The model under review builds one solid part; all positions refer to its coordinate system, in mm. Round coordinates to 2 decimals unless told otherwise and drop trailing zeros. Use CSV: the item, a comma, the result in double quotes. Start each with the question number.
1) For pin 1 Ø4 at (x, y) = (-155, 0) entering from -Z; pin 2 Ø1.5 at (y, z) = (3.5, -1) entering from +X, all flat-tipped, find the tip position at first contact; note any pin that passes through.
2) Mouldability with a two-part tool opening along Y and no side actions: class faces 1 (the face through (-2, 2, -3)), 2 (the face through (-2, -7.5, 0)), 3 (the face through (157.385, 0.751, -0.042)) as released by +Y, released by -Y, zero draft, split by the parting line, or undercut.
3) Wall thickness on probe 1 along Y at (x, z) = (-155, 0.9); probe 2 along X at (y, z) = (-1.25, 1); probe 3 along X at (y, z) = (1, 2.25): over which ranges is each line inside the solid? List them lowest first. Write a range as [from, to].
from build123d import *

# Parameters (mm, degrees)
SZKIC1_W                       = 325
SZKIC1_H                       = 15
SZKIC1_R                       = 2.5
DODANIE_WYCI_GNI_CIE1_DEPTH    = 3
ZAOKR_GLENIE1_R                = 5
OTWORY_USTALAJ_CE_3_0MM1_D     = 3
OTWORY_USTALAJ_CE_3_0MM1_DEPTH = 7.499
OTWORY_USTALAJ_CE_3_0MM1_TIP   = 0.901290929


with BuildPart() as part:
    # Szkic1 → Dodanie-wyciągnięcie1 (new, symmetric)
    with BuildSketch(Plane.XY):
        Rectangle(SZKIC1_W, SZKIC1_H)
        with Locations((155, 0)):
            Circle(SZKIC1_R, mode=Mode.SUBTRACT)
        with Locations((-155, 0)):
            Circle(SZKIC1_R, mode=Mode.SUBTRACT)
        Circle(SZKIC1_R, mode=Mode.SUBTRACT)
    extrude(amount=DODANIE_WYCI_GNI_CIE1_DEPTH, both=True)

    # Zaokrąglenie1
    zaokr_glenie1_edges = [part.edges().sort_by_distance(p)[0] for p in [
        (162.5, 7.5, 0),
        (162.5, -7.5, 0),
        (-162.5, -7.5, 0),
        (-162.5, 7.5, 0),
    ]]
    fillet(zaokr_glenie1_edges, radius=ZAOKR_GLENIE1_R)

    # Otwory ustalające Ø3.0mm1
    with Locations(Plane(origin=(0, -7.5, 0), x_dir=(-1, 0, 0), z_dir=(0, -1, 0))):
        with Locations((0, 0)):
            Hole(OTWORY_USTALAJ_CE_3_0MM1_D / 2, depth=OTWORY_USTALAJ_CE_3_0MM1_DEPTH)
            with Locations((0, 0, -(OTWORY_USTALAJ_CE_3_0MM1_DEPTH + OTWORY_USTALAJ_CE_3_0MM1_TIP / 2))):  # 118° drill point
                Cone(0, OTWORY_USTALAJ_CE_3_0MM1_D / 2, OTWORY_USTALAJ_CE_3_0MM1_TIP, mode=Mode.SUBTRACT)


solid = part.part
Values found:
1,pin 1,"through"
1,pin 2,"x = 162.49"
2,face 1,"zero draft"
2,face 2,"released by -Y"
2,face 3,"undercut"
3,probe 1,"[-7.5, -2.5], [2.5, 7.5]"
3,probe 2,"[-162.5, -157.17], [-152.83, -2.17], [2.17, 152.83], [157.17, 162.5]"
3,probe 3,"[-162.5, -157.29], [-152.71, -2.29], [2.29, 152.71], [157.29, 162.5]"
